```python
from build123d import *

# Parameters (mm, degrees)
SKETCH040_W     = 80
SKETCH040_H     = 80
PAD013_DEPTH    = 17
SKETCH041_R     = 35
POCKET014_DEPTH = 20
SKETCH044_W     = 5
SKETCH044_H     = 20.180618
POCKET017_DEPTH = 24


with BuildPart() as part:
    # Sketch040 → Pad013 (new body)
    with BuildSketch(Plane.XY):
        Rectangle(SKETCH040_W, SKETCH040_H)
    extrude(amount=-PAD013_DEPTH)

    # Sketch041 (on Face6 of Pad013) → Pocket014 (cut)
    with BuildSketch(Plane(origin=(0, 0, -17), x_dir=(1, 0, 0), z_dir=(0, 0, -1))):
        Circle(SKETCH041_R)
    extrude(amount=-POCKET014_DEPTH, mode=Mode.SUBTRACT)

    # Sketch044 (on Face5 of Pocket014) → Pocket017 (cut)
    with BuildSketch(Plane(origin=(0, 0, -17), x_dir=(1, 0, 0), z_dir=(0, 0, -1))):
        with Locations((0, -41.150577)):
            Rectangle(SKETCH044_W, SKETCH044_H)
    extrude(amount=-POCKET017_DEPTH, mode=Mode.SUBTRACT)


solid = part.part
```
Geometry check sheet. Reference: the model listing, model coordinates, mm. A direction names the side the tool comes from. Coordinates: 2 decimals unless noted, no trailing zeros. Write each loop counter-clockwise with the first axis right and the second up, starting at its lowest first coordinate (ties: lowest second). Pieces come first, ordered by that corner, then holes. Notation, with made-up numbers: M -9,17 L 2,17 A30 cw 2,44 Z; hole C -34.75,64.25 d6. An arc over 180 degrees is marked long. One line per item, written item: value. Start each with the question number.
(1) Sectioned sample at B-B, the plane x = 19.5. Enter the section's corners in (y, z).
(2) Scan lines: line 1 along X through (y, z) = (0, -3.5); line 2 along Y through (x, z) = (0, -8.25); line 3 along X through (y, z) = (12, -12). Record each from-to range of solid material in increasing order. Write a range as [from, to].
(3) Release check for a two-part mould opening along X. For faces 3 (the face through (-2.5, 37, -9)), 4 (the face through (21, 40, -8)), 5 (the face through (40, -1, -8)) record: released by +X, released by -X, zero draft, split by the parting line, or undercut.
(4) Sectioned sample at D-D, the plane x = 0. Enter the section's corners in (y, z), and give its area (3 significant figures).
(5) Tool access check on faces 1 (the face through (2.5, 37, -9)), 2 (the face through (-36, 1, 0)). Record the directions out of +Z, -Z, +X, -X, +Y, -Y that give a thin tool (end or side, any length) a straight path to the whole face; none if there is none.
(6) Sectioned sample at C-C, the plane z = -6. Enter the section's corners in (x, y), and give its area (3 significant figures).
(7) Sectioned sample at A-A, the plane y = -14. Enter the section's corners in (x, z), and give its area (3 significant figures).
Filled sheet:
1. outline: M -40,-17 L -29.06,-17 L -29.06,0 L -40,0 Z; M 29.06,-17 L 40,-17 L 40,0 L 29.06,0 Z
2. line 1: [-40, -35], [35, 40]
2. line 2: [-40, -35]
2. line 3: [-40, -32.88], [32.88, 40]
3. face 3: undercut
3. face 4: zero draft
3. face 5: released by +X
4. outline: M -40,-17 L -35,-17 L -35,0 L -40,0 Z
4. area: 85.0 mm²
5. face 1: +Z, -Z, +Y
5. face 2: +Z, +X, -X, +Y, -Y
6. outline: M -40,-40 L 40,-40 L 40,40 L 2.5,40 L 2.5,34.91 A35 cw long -2.5,34.91 L -2.5,40 L -40,40 Z
6. area: 2,530 mm²
7. outline: M -40,-17 L -32.08,-17 L -32.08,0 L -40,0 Z; M 32.08,-17 L 40,-17 L 40,0 L 32.08,0 Z
7. area: 269 mm²
